Here's how the part is built. I have some questions about the finished solid (model axes, mm). Face numbers are marked on the shaded views. A direction names the side the tool comes from. Give positions to 0.01 mm unless a question says otherwise; leave off trailing zeros. Write each loop counter-clockwise with the first axis right and the second up, starting at its lowest first coordinate (ties: lowest second). Pieces come first, ordered by that corner, then holes. Notation, with made-up numbers: M 49,14.25 L 58,14.25 A29 cw 58,46.25 Z; hole C 21.25,60.5 d4. An arc over 180 degrees is marked long. Use one line per item in the form item = value. Start each with the question number.
Autodesk Inventor part; units mm, degrees
ref_plane "YZ Plane" through (0, 0, 0) normal (1, 0, 0) x (0, 1, 0)
ref_plane "XZ Plane" through (0, 0, 0) normal (0, 1, 0) x (-1, 0, 0)
ref_plane "XY Plane" through (0, 0, 0) normal (0, 0, 1) x (1, 0, 0)
sketch "Sketch1" plane through (0, 0, 0) normal (1, 0, 0) x (0, 1, 0)
  line L0 (-6, 25) -> (6, 25)
  line L1 (6, 25) -> (6, -25)
  line L2 (6, -25) -> (-6, -25)
  line L3 (-6, -25) -> (-6, 25)
  dimension "d0" = 12
  dimension "d1" = 50
extrude "Extrusion1" add sketch "Sketch1" along normal blind 65
sketch "Sketch2" plane through (65, 0, 0) normal (1, 0, 0) x (0, 0, -1)
  line L0 (-25, 6) -> (-25, -6)
  line L1 (25, -6) -> (25, 6)
  line L2 (-25, 6) -> (25, 6)
  arc A0 (-25, 6) -> (25, 6) centre (0, 42.8137) ccw
  line L3 (-25, -6) -> (25, -6)
  line L4 (25, 3) -> (25, -6)
  line L5 (25, -6) -> (-25, -6)
  line L6 (-25, -6) -> (-25, 3)
  line L7 (0.0001, -3.2634) -> (15.0001, -3.2634)
  line L8 (15.0001, -3.2634) -> (25, 3)
  line L9 (0.0001, -3.2634) -> (-14.9999, -3.2634)
  line L10 (-14.9999, -3.2634) -> (-25, 3)
  point P0 (0, 0)
  dimension "d4" = 44.5
  dimension "d9" = 15.351
  dimension "d10" = 15.3508
extrude "Extrusion2" cut sketch "Sketch2" against normal through all contours L2 A0 | L10 L9 L7 L8 L1 L3 L0
sketch "Sketch3" plane through (65, -3.2634, -15.0001) normal (0, -1, 0) x (1, 0, 0)
  circle A0 centre (-32.5, 15) radius 15
  circle A1 centre (-32.5, 15) radius 12.5
  point P0 (-65, 15.0001)
  dimension "d14" = 25
extrude "Extrusion3" add sketch "Sketch3" along normal blind 13
sketch "Sketch4" plane through (0, 3, 25) normal (0, 0, 1) x (1, 0, 0)
  line L0 (37.7891, -20.8517) -> (27.7891, -20.8517)
  line L1 (27.7891, -20.8517) -> (27.7891, -10.8517)
  line L2 (27.7891, -10.8517) -> (37.7891, -10.8517)
  line L3 (37.7891, -10.8517) -> (37.7891, -20.8517)
  point P0 (0, -3)
  dimension "d18" = 10
  dimension "d19" = 10
extrude "Extrusion4" cut sketch "Sketch4" against normal through all
sketch "Sketch5" plane through (0, 3, 25) normal (0, 0, 1) x (1, 0, 0)
  line L0 (6, 0.5) -> (12, 0.5)
  line L1 (12, 0.5) -> (12, 2.5)
  line L2 (12, 2.5) -> (6, 2.5)
  line L3 (6, 2.5) -> (6, 0.5)
  line L4 (59, 0.5) -> (53, 0.5)
  line L5 (53, 0.5) -> (53, 2.5)
  line L6 (53, 2.5) -> (59, 2.5)
  line L7 (59, 2.5) -> (59, 0.5)
  point P0 (0, -3)
  point P1 (0, 0)
  point P2 (65, 0)
  dimension "d25" = 6
  dimension "d26" = 2
  dimension "d27" = 6
  dimension "d28" = 2
fillet "Fillet1" radius 4 2 edges at (32.5, 3, 25) (32.5, 3, -25)
fillet "Fillet2" radius 2.5 2 edges at (32.8066, -7.8517, -14.997) (32.8066, -7.8517, 14.9967)
sketch "Sketch10" plane through (65, 0, 0) normal (1, 0, 0) x (0, 0, -1)
  line L0 (-30.7469, 6.3774) -> (-5.3359, -9.5383)
  line L1 (-23.1232, 1.8245) -> (-14.9999, -3.2634)
  point P0 (0, 0)
sweep "Sweep3" cut profiles "Sketch5" path "Sketch10" path curves L0
sketch "Sketch11" plane through (65, 6, -25) normal (0, 0, -1) x (-1, 0, 0)
  line L0 (59, -0.5) -> (53, -0.5)
  line L1 (59, -0.5) -> (53, -0.5)
  line L2 (53, -0.5) -> (53, -2.5)
  line L3 (53, -2.5) -> (59, -2.5)
  line L4 (59, -2.5) -> (59, -0.5)
  line L5 (6, -0.5) -> (12, -0.5)
  line L6 (12, -0.5) -> (12, -2.5)
  line L7 (12, -2.5) -> (6, -2.5)
  line L8 (6, -2.5) -> (6, -0.5)
  point P0 (65, -6)
  point P1 (65, 0)
  point P2 (0, 0)
  dimension "d54" = 2
sketch "Sketch12" plane through (0, 0, 0) normal (-1, 0, 0) x (0, 0, 1)
  line L0 (-31.1671, 7.3521) -> (-3.1044, -10.2248)
  line L1 (-23.1233, 1.8245) -> (-15.0001, -3.2634)
  point P0 (0, 0)
sweep "Sweep4" cut profiles "Sketch11" path "Sketch12" path curves L0
properties part number "Cup_platform"
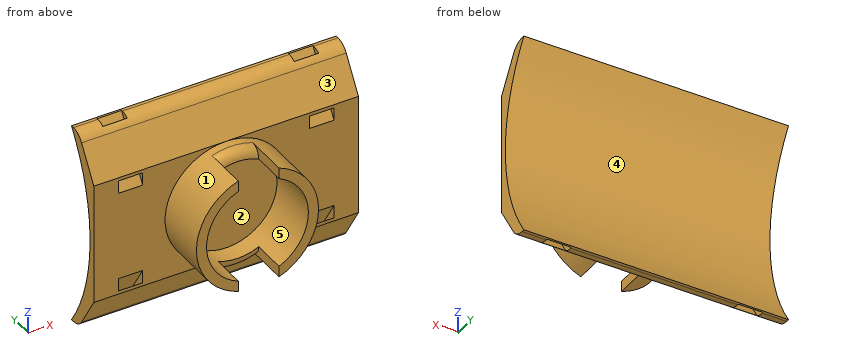
1) Will these pins go through, and if not, where does the flat tip stop? P1, Ø9.5, axis at y = 1.5, z = 15, coming from the +X side; P2, Ø2, axis at y = -12.5, z = 13, coming from the +X side; P3, Ø0.9, axis at x = 34.5, z = -12, coming from the -Y side; P4, Ø6, axis at x = 17, y = -7.5, coming from the +Z side.
2) Suppose I cut it at B-B, the plane y = -13. List the corners of the cut face in (x, z) for me.
3) On a 3-axis mill with a long thin cutter (end or side, diameter ignored), from which of +Z, -Z, +X, -X, +Y, -Y can I reach the whole of each face in a straight line? I mean the marked faces 4 and 5. Say none if no direction works.
4) Suppose I cut it at D-D, the plane x = 39. List the corners of the cut face in (y, z) for me, and give its area (3 significant figures).
5) Suppose I cut it at C-C, the plane z = 1.5. List the corners of the cut face in (x, y) for me, and give its area (3 significant figures).
6) Please list where these lines run through material, in increasing order: line 1 (X direction, y = -0.5, z = 16); line 2 (X direction, y = -5.75, z = 8); line 3 (Z direction, x = 22, y = 2.5).
7) Thinking about a two-plate mould opening in X: for the marked faces 1, 2 and 3, which applies, released by +X, released by -X, zero draft, split by the parting line, or undercut?
8) Suppose I cut it at A-A, the plane y = 0. List the corners of the cut face in (x, z) for me, and give its area (3 significant figures).
Checks:
q1.P1 = 65
q1.P2 = 41.5
q1.P3 = -7.85
q1.P4 = 8.29
q2.outline = M 27.79,-14.24 L 27.79,-11.58 A12.5 cw 27.79,11.58 L 27.79,14.24 A15 ccw Z; M 37.79,-14.04 A15 ccw 37.79,14.04 L 37.79,11.33 A12.5 cw 37.79,-11.33 Z
q3.face_4 = +X, -X, +Y
q3.face_5 = -Y
q4.outline = M -16.26,-13.52 L -3.26,-13.52 L -3.26,-15 L 1.82,-23.12 A4 ccw 5.21,-25 L 6,-25 A44.5 cw 6,25 L 5.21,25 A4 ccw 1.82,23.12 L -3.26,15 L -3.26,13.52 L -16.26,13.52 L -16.26,10.68 L -3.26,10.68 L -3.26,-10.68 L -16.26,-10.68 Z
q4.area = 212 mm^2
q5.outline = M 0,-3.26 L 17.58,-3.26 L 17.58,-16.26 L 20.09,-16.26 L 20.09,-3.26 L 44.91,-3.26 L 44.91,-16.26 L 47.42,-16.26 L 47.42,-3.26 L 65,-3.26 L 65,-1.66 L 0,-1.66 Z
q5.area = 170 mm^2
q6.line_1 = 0 to 6, 12 to 53, 59 to 65
q6.line_2 = 19.81 to 22.9, 42.1 to 45.19
q6.line_3 = -23.94 to -18.84, 18.84 to 23.94
q7.face_1 = split by the parting line
q7.face_2 = undercut
q7.face_3 = zero draft
q8.outline = M 0,-20.21 L 65,-20.21 L 65,-12.13 L 0,-12.13 Z; M 0,12.13 L 65,12.13 L 65,20.21 L 0,20.21 Z; hole M 6,-19.41 L 12,-19.41 L 12,-16.22 L 6,-16.22 Z; hole M 6,16.22 L 12,16.22 L 12,19.41 L 6,19.41 Z; hole M 53,-19.41 L 59,-19.41 L 59,-16.22 L 53,-16.22 Z; hole M 53,16.22 L 59,16.22 L 59,19.41 L 53,19.41 Z
q8.area = 973 mm^2
